Answer from the drawing. Dimensions are ordinates in mm from the lowest x, y and z of the part. Coordinates: 2 decimals unless noted, no trailing zeros. Write each loop counter-clockwise with the first axis right and the second up, starting at its lowest first coordinate (ties: lowest second). Pieces come first, ordered by that corner, then holes. Notation, with made-up numbers: (13.5, -36) -> (47.5, -36) arc R16 cw to (47.5, -11) -> close; hole circle Ø8 at (70, 10). An arc over 180 degrees is marked (long way). One line per item, written item: value. Start each with the question number.
1. Find section A-A, the plane z = 22.5. State how many separate pieces and enclosed holes the cut face has, and give its area (3 significant figures).
2. Find section D-D, the plane x = 7.5. Write down the section's boundary in (y, z), and give its area (3 significant figures).
3. For a pull along X with two mould halves and no side action, classify the marked faces 1, 2, 3 and 4 as pulls with the +X half, pulls with the -X half, needs draft (parallel to the pull), parting line crosses it, or undercut.
4. Consider line 1 along X through (y, z) = (1.8, 22.5); line 2 along X through (y, z) = (13, 22.5); line 3 along Z through (x, y) = (42, 3.5) (1 decimal). Determine where each line is inside the solid, lowest interval first.
5. Find section C-C, the plane y = 18. Write down the section's boundary in (x, z).
6. Given P1, Ø6, axis at y = 23, z = 29.5, coming from the +X side; P2, Ø10, axis at y = 13.5, z = 25.5, coming from the -X side; P3, Ø4, axis at x = 49, z = 20, coming from the +Y side; P4, Ø6.5, axis at x = 62.5, z = 22.5, coming from the -Y side (3 decimals), each flat-ended and moving along its own axis, determine where each tip first touches the part or whether it passes through.
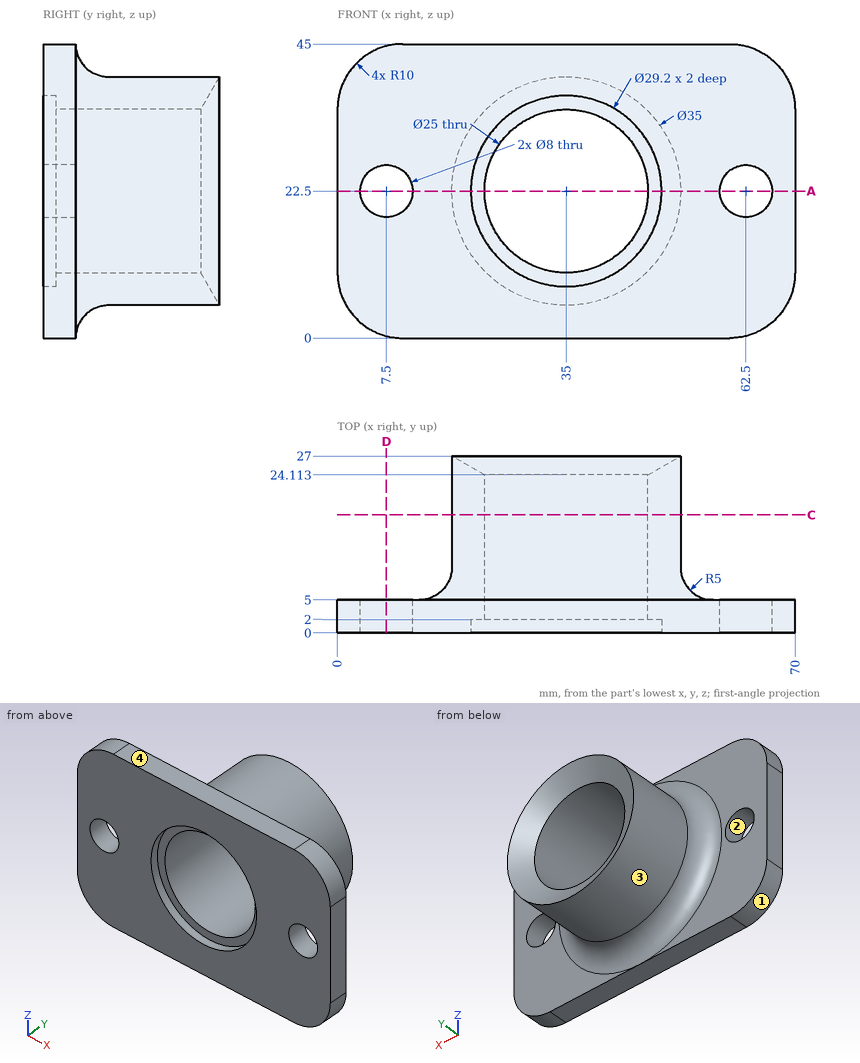
Answer block:
1. separate pieces: 4
1. enclosed holes: 0
1. area: 353 mm2
2. outline: (0, 0.32) -> (5, 0.32) -> (5, 18.5) -> (0, 18.5) -> close; (0, 26.5) -> (5, 26.5) -> (5, 44.68) -> (0, 44.68) -> close
2. area: 182 mm2
3. face 1: pulls with the -X half
3. face 2: undercut
3. face 3: parting line crosses it
3. face 4: needs draft
4. line 1: x = 0 to 3.5, 11.5 to 20.4, 49.6 to 58.5, 66.5 to 70
4. line 2: x = 17.5 to 22.5, 47.5 to 52.5
4. line 3: z = 0 to 12.1, 32.9 to 45
5. outline: circle Ø35 at (35, 22.5); hole circle Ø25 at (35, 22.5)
6. P1: stops at x = 52.04
6. P2: stops at x = 17.4
6. P3: stops at y = 26.26
6. P4: passes through
